from build123d import *

# Parameters (mm, degrees)
BOSS_EXTRU_1_DEPTH      = 7
ESQUISSE2_R             = 3
ENL_V_MAT_EXTRU_1_DEPTH = 7
ESQUISSE3_R             = 1.6
ENL_V_MAT_EXTRU_2_DEPTH = 7
ESQUISSE5_R             = 12.5
ENL_V_MAT_EXTRU_5_DEPTH = 5
ESQUISSE17_R            = 6
ESQUISSE17_R_2          = 4
BOSS_EXTRU_6_DEPTH      = 3.5
BOSS_EXTRU_8_DEPTH      = 8
ENL_V_START             = -8
ESQUISSE19_R            = 4
ENL_V_MAT_EXTRU_6_DEPTH = 8


with BuildPart() as part:
    # Esquisse1 → Boss.-Extru.1 (new body)
    with BuildSketch(Plane.XY):
        with BuildLine():
            Line((9, 0), (16, -50))
            ThreePointArc((16, -50), (0, -66), (-16, -50))
            Line((-16, -50), (-9, 0))
            ThreePointArc((-9, 0), (0, 9), (9, 0))
        make_face()
    extrude(amount=BOSS_EXTRU_1_DEPTH)

    # Esquisse2 → Enlèv. mat.-Extru.1 (cut)
    with BuildSketch(Plane.XY.offset(7)):
        with Locations((0, -50)):
            Circle(ESQUISSE2_R)
    extrude(amount=-ENL_V_MAT_EXTRU_1_DEPTH, mode=Mode.SUBTRACT)

    # Esquisse3 → Enlèv. mat.-Extru.2 (cut)
    with BuildSketch(Plane.XY.offset(7)):
        with Locations((0, -59)):
            Circle(ESQUISSE3_R)
        with Locations((-7.794228634, -45.5)):
            Circle(ESQUISSE3_R)
        with Locations((7.794228634, -45.5)):
            Circle(ESQUISSE3_R)
    extrude(amount=-ENL_V_MAT_EXTRU_2_DEPTH, mode=Mode.SUBTRACT)

    # Esquisse5 → Enlèv. mat.-Extru.5 (cut)
    with BuildSketch(Plane.XY.offset(7)):
        with Locations((0, -50)):
            Circle(ESQUISSE5_R)
    extrude(amount=-ENL_V_MAT_EXTRU_5_DEPTH, mode=Mode.SUBTRACT)

    # Esquisse17 → Boss.-Extru.6 (add)
    with BuildSketch(Plane.XY.offset(7)):
        with Locations(Location((0, 0, 0), (0, 0, 180))):
            Circle(ESQUISSE17_R)
        Circle(ESQUISSE17_R_2, mode=Mode.SUBTRACT)
    extrude(amount=BOSS_EXTRU_6_DEPTH)

    # Esquisse18 → Boss.-Extru.8 (add)
    with BuildSketch(Plane.XY.offset(7)):
        with BuildLine():
            Line((-10.825317547, -43.75), (-13.856406461, -42))
            ThreePointArc((-13.856406461, -42), (-14.731391476, -43.756114576), (-15.384856807, -45.606120047))
            Line((-15.384856807, -45.606120047), (-16, -50))
            ThreePointArc((-16, -50), (0, -66), (16, -50))
            Line((16, -50), (15.384856807, -45.606120047))
            ThreePointArc((15.384856807, -45.606120047), (14.731391476, -43.756114576), (13.856406461, -42))
            Line((13.856406461, -42), (10.825317547, -43.75))
            ThreePointArc((10.825317547, -43.75), (12.074072829, -46.764761936), (12.5, -50))
            ThreePointArc((12.5, -50), (-3.235238064, -62.074072829), (-10.825317547, -43.75))
        make_face()
    extrude(amount=BOSS_EXTRU_8_DEPTH)

    # Esquisse19 → Enlèv. mat.-Extru.6 (cut)
    with BuildSketch(Plane.XY.offset(7).offset(ENL_V_START)):
        with Locations(Location((0, 0, 0), (0, 0, 180))):
            Circle(ESQUISSE19_R)
    extrude(amount=ENL_V_MAT_EXTRU_6_DEPTH, mode=Mode.SUBTRACT)


solid = part.part
Work out the finished part from the listing and answer in its coordinate system (mm). A direction names the side the tool comes from. Give positions to 0.01 mm unless a question says otherwise; leave off trailing zeros. Loops run counter-clockwise (first coordinate to the right, second up) from the corner with the lowest first, then second, coordinate; pieces in that order, holes last. Notation, with made-up numbers: (8, 14.5) - (41, 14.5) arc R25 ccw to (41, 36.5) - close; hole circle Ø7 at (-16, 43). An arc over 180 degrees is marked (long way). Answer in a Markdown table with one row per item.
(1) Section C-C (y = -59) is taken. Give the vertices of the cut face in (x, z), and give its area (3 significant figures).
Results list:
| item | result |
|---|---|
| outline | (-13.23, 0) - (-1.6, 0) - (-1.6, 2) - (-8.67, 2) - (-8.67, 15) - (-13.23, 15) - close; (1.6, 0) - (13.23, 0) - (13.23, 15) - (8.67, 15) - (8.67, 2) - (1.6, 2) - close |
| area | 165 mm² |
(2) A tool of negligible diameter and unlimited length cuts with its end or side. For faces 1 (the face through (3, -53, 2)), 2 (the face through (0, -66, 7)), 3 (the face through (12.362, -42.863, 10.944)), 4 (the face through (-14.72, -43.73, 10.94)), 5 (the face through (14.74, -43.78, 10.94)), from which of +Z, -Z, +X, -X, +Y, -Y can it reach the whole face along a straight path? Write none if from no direction.
Results list:
| item | result |
|---|---|
| face 1 | +Z |
| face 2 | +Z, -Z, -Y |
| face 3 | +Z, +Y |
| face 4 | +Z, -X, +Y |
| face 5 | +Z, +X, +Y |
(3) Section B-B (x = 0) is taken. Give the vertices of the cut face in (y, z).
Results list:
| item | result |
|---|---|
| outline | (-66, 0) - (-60.6, 0) - (-60.6, 2) - (-62.5, 2) - (-62.5, 15) - (-66, 15) - close; (-57.4, 0) - (-53, 0) - (-53, 2) - (-57.4, 2) - close; (-47, 0) - (-4, 0) - (-4, 10.5) - (-6, 10.5) - (-6, 7) - (-37.5, 7) - (-37.5, 2) - (-47, 2) - close; (4, 0) - (9, 0) - (9, 7) - (6, 7) - (6, 10.5) - (4, 10.5) - close |
(4) For a pull along Y with two mould halves and no side action, classify faces 6 (the face through (-12.3, -42.9, 10.9)), 7 (the face through (0, -24, 7)), 8 (the face through (-3.92, -1.42, 10.5)) as pulls with the +Y half, pulls with the -Y half, needs draft (parallel to the pull), parting line crosses it, or undercut.
Results list:
| item | result |
|---|---|
| face 6 | pulls with the +Y half |
| face 7 | undercut |
| face 8 | needs draft |
(5) Consider L1, parallel to Y at x = 0, z = 1.5; L2, parallel to Y at x = 0, z = 3.5; L3, parallel to Z at x = -4.5, y = -9. Determine where each line is inside the solid, lowest interval first. Write a range as [from, to].
Results list:
| item | result |
|---|---|
| L1 | y = [-66, -60.6], [-57.4, -53], [-47, -4], [4, 9] |
| L2 | y = [-66, -62.5], [-37.5, -4], [4, 9] |
| L3 | z = [0, 7] |
(6) Flat-ended cylindrical pins translate along their axes: pin 1 Ø8 at (x, y) = (-9.5, -30) entering from +Z; pin 2 Ø3.5 at (x, y) = (0, -59) entering from +Z; pin 3 Ø3 at (x, z) = (5, 9.5) entering from +Y. Find the tip coordinate at first contact, or state that the pin passes through.
Results list:
| item | result |
|---|---|
| pin 1 | stops at z = 7 |
| pin 2 | stops at z = 2 |
| pin 3 | stops at y = 4.87 |
(7) Section A-A (z = 9.75) is taken. Give the vertices of the cut face in (x, y).
Results list:
| item | result |
|---|---|
| outline | (-16, -50) arc R16 ccw to (16, -50) - (15.38, -45.61) arc R16 ccw to (13.86, -42) - (10.83, -43.75) arc R12.5 cw (long way) to (-10.83, -43.75) - (-13.86, -42) arc R16 ccw to (-15.38, -45.61) - close; circle Ø12 at (0, 0); hole circle Ø8 at (0, 0) |
(8) Section D-D (x = 8) is taken. Give the vertices of the cut face in (y, z).
Results list:
| item | result |
|---|---|
| outline | (-63.86, 0) - (-47.09, 0) - (-47.09, 2) - (-59.6, 2) - (-59.6, 15) - (-63.86, 15) - close; (-43.91, 0) - (4.12, 0) - (4.12, 7) - (-40.4, 7) - (-40.4, 2) - (-43.91, 2) - close |
